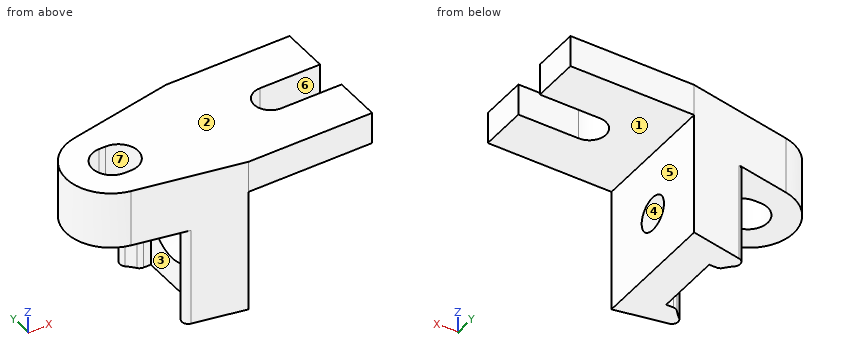
from build123d import *

# Parameters (mm, degrees)
PAD_DEPTH       = 24.5
SKETCH001_W     = 15
SKETCH001_H     = 12
POCKET_DEPTH    = 14.5
SKETCH002_W     = 20
SKETCH002_H     = 20
POCKET001_DEPTH = 19.5
SKETCH003_R     = 2.7
POCKET002_DEPTH = 22.19959
POCKET003_DEPTH = 15.5
CHAMFER_SIZE    = 2.4
FILLET_R        = 1


with BuildPart() as part:
    # Sketch → Pad (new body)
    with BuildSketch(Plane.XY):
        with BuildLine():
            Line((-2, 6.87796), (14.5, 10))
            Line((14.5, 10), (34, 10))
            Line((34, 10), (34, 2.6))
            Line((24.5, 2.6), (34, 2.6))
            ThreePointArc((24.5, 2.6), (21.9, 0), (24.5, -2.6))
            Line((24.5, -2.6), (34, -2.6))
            Line((34, -2.6), (34, -10))
            Line((34, -10), (14.5, -10))
            Line((14.5, -10), (-2, -6.87796))
            ThreePointArc((-2, 6.87796), (-7.69859, 0), (-2, -6.87796))
        make_face()
        with BuildLine():
            ThreePointArc((-0.5, 3.1), (-3.6, 0), (-0.5, -3.1))
            Line((-0.5, -3.1), (0.5, -3.1))
            ThreePointArc((0.5, -3.1), (3.6, 0), (0.5, 3.1))
            Line((-0.5, 3.1), (0.5, 3.1))
        make_face(mode=Mode.SUBTRACT)
    extrude(amount=PAD_DEPTH)

    # Sketch001 (on Face3 of Pad) → Pocket (cut)
    with BuildSketch(Plane.YZ.offset(34)):
        with Locations((2, 0)):
            Rectangle(SKETCH001_W, SKETCH001_H)
    extrude(amount=-POCKET_DEPTH, mode=Mode.SUBTRACT)

    # Sketch002 (on Face4 of Pocket) → Pocket001 (cut)
    with BuildSketch(Plane(origin=(0, 0, 0), x_dir=(1, 0, 0), z_dir=(0, 0, -1))):
        with Locations((24.5, 0)):
            Rectangle(SKETCH002_W, SKETCH002_H)
    extrude(amount=-POCKET001_DEPTH, mode=Mode.SUBTRACT)

    # Sketch003 (on Face5 of Pocket001) → Pocket002 (cut, through all)
    with BuildSketch(Plane.YZ.offset(14.5)):
        with Locations((0, 9.5)):
            Circle(SKETCH003_R)
    extrude(amount=-POCKET002_DEPTH, mode=Mode.SUBTRACT)

    # Sketch004 (on Face2 of Pocket002) → Pocket003 (cut)
    with BuildSketch(Plane(origin=(0, 0, 0), x_dir=(1, 0, 0), z_dir=(0, 0, -1))):
        with BuildLine():
            ThreePointArc((7.345747, 5.2), (-9, 0), (7.345747, -5.2))
            Line((9, -5.2), (7.345747, -5.2))
            Line((9, 5.2), (9, -5.2))
            Line((7.345747, 5.2), (9, 5.2))
        make_face()
    extrude(amount=-POCKET003_DEPTH, mode=Mode.SUBTRACT)

    # Chamfer
    chamfer_edges = [part.edges().sort_by_distance(p)[0] for p in [
        (9, -2.7, 9.5),
    ]]
    chamfer(chamfer_edges, length=CHAMFER_SIZE)

    # Fillet
    fillet_edges = [part.edges().sort_by_distance(p)[0] for p in [
        (4.070941, 8.02667, 7.75),
        (7.345747, 5.2, 7.75),
        (7.345747, -5.2, 7.75),
        (4.070941, -8.02667, 7.75),
    ]]
    fillet(fillet_edges, radius=FILLET_R)


solid = part.part
Source: CAD feature listing. Evaluate the final solid. Frame: model axes, mm. Face numbers are marked on the shaded views. A direction names the side the tool comes from. Give positions to 0.01 mm unless a question says otherwise; leave off trailing zeros. Write each loop counter-clockwise with the first axis right and the second up, starting at its lowest first coordinate (ties: lowest second). Pieces come first, ordered by that corner, then holes. Notation, with made-up numbers: (68, 31) -> (110, 31) arc R26 cw to (110, 61) -> close; hole circle Ø3 at (18.5, -40). An arc over 180 degrees is marked (long way). Return JSON: item names as keys, results as strings. Group by question number.
1. Section C-C, the plane z = 9.5. Output: boundary loops of the cut face in (x, y), then the cut area to 3 significant figures.
2. Material intervals for line 1 (Z direction, x = 13.6, y = 0); line 2 (Z direction, x = 5, y = 8); line 3 (Z direction, x = 30, y = -3), sorted ascending. Write a range as from..to.
3. Section B-B, the plane z = 21. Output: boundary loops of the cut face in (x, y), then the cut area to 3 significant figures.
4. Pin query (flat end, axial travel): pin 1 Ø11.5 at (y, z) = (-1.5, 10.5) entering from -X; pin 2 Ø1.1 at (x, z) = (0, 22) entering from -Y; pin 3 Ø1.3 at (x, z) = (8.5, 9.5) entering from -Y; pin 4 Ø1.3 at (x, z) = (8.5, 4) entering from +Y. Return the tip coordinate at first contact, or that it passes through.
5. Mould query, pull axis Z, two halves, no side actions, for the marked faces 1, 2, 3 and 4. Classes: +Z half, -Z half, draft (parallel to the pull), parting line (faces both ways), or undercut.
6. Access query for the marked faces 5, 6 and 7. Directions: +Z, -Z, +X, -X, +Y, -Y. A direction counts if a zero-diameter tool reaches every point of the face in a straight line with its end or side. Return the directions, or none.
7. Section D-D, the plane y = 6.25. Output: boundary loops of the cut face in (x, z), then the cut area to 3 significant figures.
8. Section A-A, the plane x = 31.5. Output: boundary loops of the cut face in (y, z), then the cut area to 3 significant figures.
Determined:
{
 "1": {"outline": "(5.96, -6.74) arc R1 ccw to (6.44, -8.47) -> (14.5, -10) -> (14.5, -2.7) -> (11.4, -2.7) -> (9, -5.1) -> (9, -5.2) -> (7.85, -5.2) arc R1 ccw to (7.06, -5.58) arc R9 cw to start; (5.96, 6.74) arc R9 cw to (7.06, 5.58) arc R1 ccw to (7.85, 5.2) -> (9, 5.2) -> (9, 5.1) -> (11.4, 2.7) -> (14.5, 2.7) -> (14.5, 10) -> (6.44, 8.47) arc R1 ccw to start", "area": "88.2 mm2"},
 "2": {"line 1": "z = 0..6.8, 12.2..24.5", "line 2": "z = 15.5..24.5", "line 3": "z = 19.5..24.5"},
 "3": {"outline": "(-2, -6.88) -> (14.5, -10) -> (34, -10) -> (34, -2.6) -> (24.5, -2.6) arc R2.6 cw to (24.5, 2.6) -> (34, 2.6) -> (34, 10) -> (14.5, 10) -> (-2, 6.88) arc R7 ccw to start; hole (-0.5, -3.1) -> (0.5, -3.1) arc R3.1 ccw to (0.5, 3.1) -> (-0.5, 3.1) arc R3.1 ccw to start", "area": "631 mm2"},
 "4": {"pin 1": "stops at x = -7.7", "pin 2": "stops at y = -7.36", "pin 3": "stops at y = -8.99", "pin 4": "stops at y = 8.99"},
 "5": {"face 1": "-Z half", "face 2": "+Z half", "face 3": "draft", "face 4": "undercut"},
 "6": {"face 5": "-Z, +X, +Y, -Y", "face 6": "+Z, -Z, +X", "face 7": "+Z, -Z"},
 "7": {"outline": "(-3.85, 15.5) -> (6.48, 15.5) -> (6.48, 0) -> (14.5, 0) -> (14.5, 19.5) -> (34, 19.5) -> (34, 24.5) -> (-3.85, 24.5) -> close", "area": "387 mm2"},
 "8": {"outline": "(-10, 19.5) -> (-2.6, 19.5) -> (-2.6, 24.5) -> (-10, 24.5) -> close; (2.6, 19.5) -> (10, 19.5) -> (10, 24.5) -> (2.6, 24.5) -> close", "area": "74.0 mm2"}
}
